```python
from build123d import *

# Parameters (mm, degrees)
PAD_DEPTH       = 16
SKETCH001_R     = 2.15
SKETCH001_W     = 2.6
SKETCH001_H     = 6
POCKET_DEPTH    = 43.001
SKETCH002_R     = 2.15
POCKET001_DEPTH = 8
SKETCH003_R     = 2.15
POCKET002_DEPTH = 8
CHAMFER_SIZE    = 1


with BuildPart() as part:
    # Sketch → Pad (new body)
    with BuildSketch(Plane.XY):
        Polygon((0, 0), (0, 43), (76.6, 43), (76.6, 31), (152.2, 31), (152.2, 0), align=None)
    extrude(amount=PAD_DEPTH)

    # Sketch001 → Pocket (cut, through all)
    with BuildSketch(Plane.XZ):
        with Locations((12, 8)):
            Circle(SKETCH001_R)
        with Locations((89.6, 8)):
            Circle(SKETCH001_R)
        with Locations((140.2, 8)):
            Circle(SKETCH001_R)
        with Locations((57.6, 8)):
            Circle(SKETCH001_R)
        with Locations((21.3, 3)):
            Rectangle(SKETCH001_W, SKETCH001_H)
        with Locations((130.9, 3)):
            Rectangle(SKETCH001_W, SKETCH001_H)
    extrude(amount=-POCKET_DEPTH, mode=Mode.SUBTRACT)

    # Sketch002 → Pocket001 (cut)
    with BuildSketch(Plane.YZ):
        with Locations((12, 8)):
            Circle(SKETCH002_R)
    extrude(amount=POCKET001_DEPTH, mode=Mode.SUBTRACT)

    # Sketch003 (on DatumPlane) → Pocket002 (cut)
    with BuildSketch(Plane.YZ.offset(152.2)):
        with Locations((12, 8)):
            Circle(SKETCH003_R)
    extrude(amount=-POCKET002_DEPTH, mode=Mode.SUBTRACT)

    # Chamfer
    chamfer_edges = [part.edges().sort_by_distance(p)[0] for p in [
        (0, 9.85, 8),
        (9.85, 0, 8),
        (55.45, 0, 8),
        (87.45, 0, 8),
        (138.05, 0, 8),
        (152.2, 9.85, 8),
        (138.05, 31, 8),
        (87.45, 31, 8),
        (55.45, 43, 8),
        (9.85, 43, 8),
    ]]
    chamfer(chamfer_edges, length=CHAMFER_SIZE)


solid = part.part
```
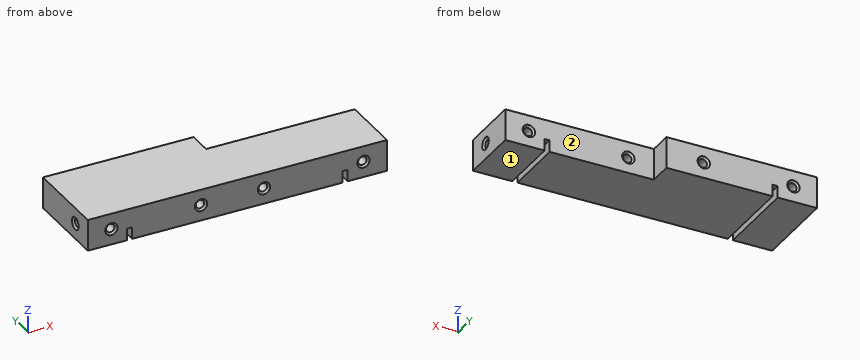
Could you check a few things on this model? Use its own coordinates, in mm. Face numbers are marked on the shaded views. A direction names the side the tool comes from. Round coordinates to 2 decimals unless told otherwise and drop trailing zeros. Write each loop counter-clockwise with the first axis right and the second up, starting at its lowest first coordinate (ties: lowest second). Pieces come first, ordered by that corner, then holes. Notation, with made-up numbers: M -5.75,-27 L 14.25,-27 A20 cw 14.25,-16 Z; hole C 39.25,-7.5 d1. An arc over 180 degrees is marked long. Answer in a Markdown table with one row per item. Add a question column.
Q1. Imagine slicing it at B-B (x = 89.6). Please give me the cut outline in (y, z), then the cut area to 3 significant figures.
Q2. Will these pins go through, and if not, where does the flat tip stop? pin 1 Ø4 at (x, z) = (89.6, 8) entering from -Y; pin 2 Ø1.5 at (x, z) = (58.5, 10) entering from +Y; pin 3 Ø4.5 at (y, z) = (12.5, 7.5) entering from +X; pin 4 Ø1.3 at (x, y) = (131, 13.5) entering from -Z.
Q3. Imagine slicing it at D-D (z = 8). Give the number of separate pieces and of enclosed holes in the cut face, then the cut area to 3 significant figures.
Q4. Imagine slicing it at C-C (y = 22). Please give me the cut outline in (x, z).
Q5. If I drill on line 1 (X direction, y = 27.5, z = 8.25); line 2 (Z direction, x = 57.6, y = 32); line 3 (X direction, y = 6, z = 1.75), over which ranges is the centre line in solid material (lowest first)? Write a range as from..to.
Q6. On a 3-axis mill with a long thin cutter (end or side, diameter ignored), from which of +Z, -Z, +X, -X, +Y, -Y can I reach the whole of each face in a straight line? I mean the marked faces 1 and 2. Say none if no direction works.
Q7. Imagine slicing it at A-A (z = 2). Please give me the cut outline in (x, y).
Values:
| question | item | result |
|---|---|---|
| 1 | outline | M 0,0 L 31,0 L 31,4.85 L 30,5.85 L 1,5.85 L 0,4.85 Z; M 0,11.15 L 1,10.15 L 30,10.15 L 31,11.15 L 31,16 L 0,16 Z |
| 1 | area | 361 mm^2 |
| 2 | pin 1 | through |
| 2 | pin 2 | y = 42.79 |
| 2 | pin 3 | x = 152.01 |
| 2 | pin 4 | z = 6 |
| 3 | separate pieces | 5 |
| 3 | enclosed holes | 0 |
| 3 | area | 4,920 mm^2 |
| 4 | outline | M 0,0 L 20,0 L 20,6 L 22.6,6 L 22.6,0 L 129.6,0 L 129.6,6 L 132.2,6 L 132.2,0 L 152.2,0 L 152.2,16 L 0,16 Z; hole C 12,8 d4.3; hole C 57.6,8 d4.3; hole C 89.6,8 d4.3; hole C 140.2,8 d4.3 |
| 5 | line 1 | 0..9.86, 14.14..55.46, 59.74..87.46, 91.74..138.06, 142.34..152.2 |
| 5 | line 2 | 0..5.85, 10.15..16 |
| 5 | line 3 | 0..20, 22.6..129.6, 132.2..152.2 |
| 6 | face 1 | -Z, +X, -X, +Y, -Y |
| 6 | face 2 | +Z, -Z, +X, +Y |
| 7 | outline | M 0,0 L 20,0 L 20,43 L 0,43 Z; M 22.6,0 L 129.6,0 L 129.6,31 L 76.6,31 L 76.6,43 L 22.6,43 Z; M 132.2,0 L 152.2,0 L 152.2,31 L 132.2,31 Z |
